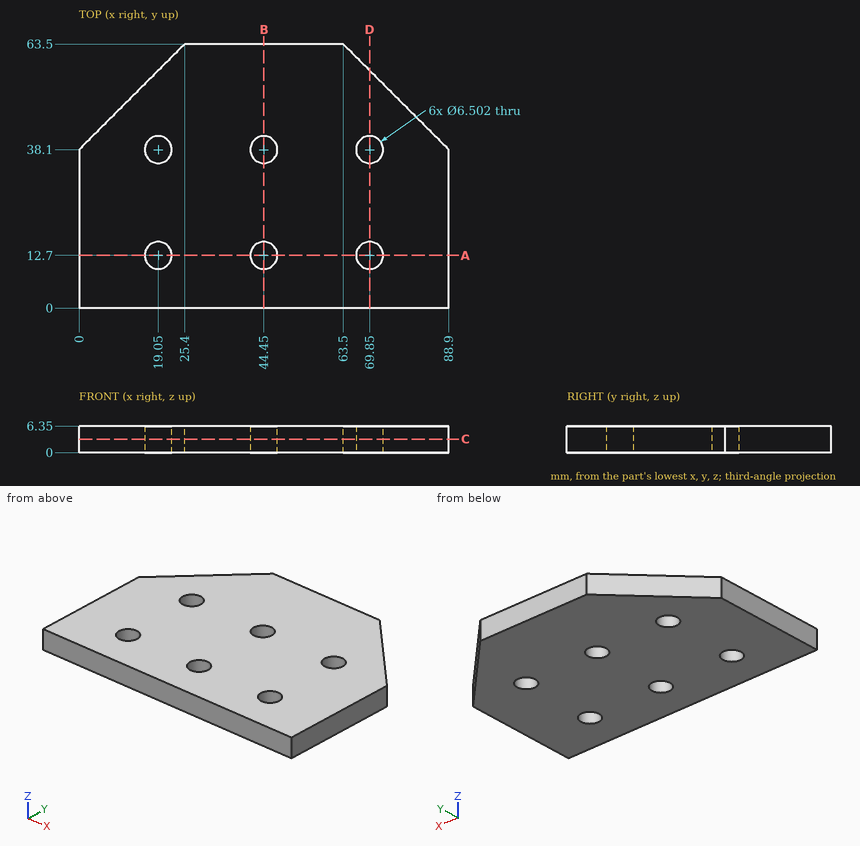
Part print with two shaded views. Sizes in mm from the minimum x, y, z corner. Give positions to 0.01 mm unless a question says otherwise; leave off trailing zeros. Order: outer loops, then holes, each group sorted by start corner. A loop starts at its lowest first (then second) coordinate and runs counter-clockwise, first axis right, second up. Notation, with made-up numbers: (-16, 8) - (41, 8) arc R14 cw to (41, 32) - close; hole circle Ø9 at (-21.5, -10). An arc over 180 degrees is marked (long way). Write each question's results on one line, items separated by ' | '.
1. Saw through at A-A on y = 12.7. List the corners of the cut face in (x, z).
Calculated:
outline: (0, 0) - (15.8, 0) - (15.8, 6.35) - (0, 6.35) - close; (22.3, 0) - (41.2, 0) - (41.2, 6.35) - (22.3, 6.35) - close; (47.7, 0) - (66.6, 0) - (66.6, 6.35) - (47.7, 6.35) - close; (73.1, 0) - (88.9, 0) - (88.9, 6.35) - (73.1, 6.35) - close
2. Saw through at D-D on x = 69.85. List the corners of the cut face in (y, z).
Calculated:
outline: (0, 0) - (9.45, 0) - (9.45, 6.35) - (0, 6.35) - close; (15.95, 0) - (34.85, 0) - (34.85, 6.35) - (15.95, 6.35) - close; (41.35, 0) - (57.15, 0) - (57.15, 6.35) - (41.35, 6.35) - close
3. Probe L1, parallel to X at y = 11, z = 4; L2, parallel to X at y = 41, z = 1.5; L3, parallel to Y at x = 72, z = 0.5. List the from-to ranges inside material, lowest first. Write a range as from..to.
Calculated:
L1: x = 0..16.28, 21.82..41.68, 47.22..67.08, 72.62..88.9 | L2: x = 2.9..17.58, 20.52..42.98, 45.92..68.38, 71.32..86 | L3: y = 0..10.26, 15.14..35.66, 40.54..55
4. Pin check, flat tip, straight feed: pin 1 (6 mm diameter, centred on x = 69.85, y = 12.7, fed in from +Z). Stop position of the tip, or through.
Calculated:
pin 1: passes through
5. Saw through at B-B on x = 44.45. List the corners of the cut face in (y, z), and give its area (3 significant figures).
Calculated:
outline: (0, 0) - (9.45, 0) - (9.45, 6.35) - (0, 6.35) - close; (15.95, 0) - (34.85, 0) - (34.85, 6.35) - (15.95, 6.35) - close; (41.35, 0) - (63.5, 0) - (63.5, 6.35) - (41.35, 6.35) - close | area: 321 mm2
6. Saw through at C-C on z = 3.25. List the corners of the cut face in (x, y), and give its area (3 significant figures).
Calculated:
outline: (0, 0) - (88.9, 0) - (88.9, 38.1) - (63.5, 63.5) - (25.4, 63.5) - (0, 38.1) - close; hole circle Ø6.5 at (19.05, 12.7); hole circle Ø6.5 at (19.05, 38.1); hole circle Ø6.5 at (44.45, 12.7); hole circle Ø6.5 at (44.45, 38.1); hole circle Ø6.5 at (69.85, 12.7); hole circle Ø6.5 at (69.85, 38.1) | area: 4,800 mm2
